The listing builds one solid part. Answer for the finished solid, in the listing's coordinates (mm). A direction names the side the tool comes from. Coordinates: 2 decimals unless noted, no trailing zeros. Loops run counter-clockwise (first coordinate to the right, second up) from the corner with the lowest first, then second, coordinate; pieces in that order, holes last. Notation, with made-up numbers: (-5, 83.5) - (12, 83.5) arc R25 cw to (12, 106.5) - close; hole circle Ø5 at (23.5, 25.5). An arc over 180 degrees is marked (long way). Put each result on its own line as item: value.
```python
from build123d import *

# Parameters (mm, degrees)
SKETCH2_R           = 1.6
CUT_EXTRUDE1_DEPTH  = 62.102373113
SKETCH8_R           = 10
CUT_EXTRUDE6_DEPTH  = 2
SKETCH16_R          = 1.5
CUT_EXTRUDE7_DEPTH  = 4
CUT_EXTRUDE10_DEPTH = 2


with BuildPart() as part:
    # Sketch1 → Revolve1 (revolve)
    with BuildSketch(Plane(origin=(0, 0, 0), x_dir=(0, 0, -1), z_dir=(1, 0, 0)), mode=Mode.PRIVATE) as revolve1_sk:
        Polygon((0, 0), (0, 42.5), (-3, 42.5), (-3, 19.55), (-3.5, 19.55), (-3.5, 17.55), (-11, 17.55), (-11, 0), align=None)
    revolve(revolve1_sk.sketch.rotate(Axis((0, 0, 11), (0, 0, -1)), 90), axis=Axis((0, 0, 11), (0, 0, -1)))

    # Sketch2 → Cut-Extrude1 (cut, through all)
    with BuildSketch(Plane(origin=(0, 0, 0), x_dir=(-1, 0, 0), z_dir=(0, 0, -1))):
        with Locations(Location((0, 36.75, 0), (0, 0, 90))):
            Circle(SKETCH2_R)
        with Locations(Location((36.75, 0, 0), (0, 0, 90))):
            Circle(SKETCH2_R)
        with Locations(Location((0, -36.75, 0), (0, 0, 90))):
            Circle(SKETCH2_R)
        with Locations(Location((-36.75, 0, 0), (0, 0, 90))):
            Circle(SKETCH2_R)
    extrude(amount=-CUT_EXTRUDE1_DEPTH, mode=Mode.SUBTRACT)

    # Sketch8 → Cut-Extrude6 (cut)
    with BuildSketch(Plane(origin=(0, 0, 0), x_dir=(-1, 0, 0), z_dir=(0, 0, -1))):
        Circle(SKETCH8_R)
    extrude(amount=-CUT_EXTRUDE6_DEPTH, mode=Mode.SUBTRACT)

    # Sketch16 → Cut-Extrude7 (cut)
    with BuildSketch(Plane(origin=(0, 0, 2), x_dir=(-1, 0, 0), z_dir=(0, 0, -1))):
        with Locations((4.065863992, 4.065863992)):
            Circle(SKETCH16_R)
        with Locations((-4.065863992, -4.065863992)):
            Circle(SKETCH16_R)
    extrude(amount=-CUT_EXTRUDE7_DEPTH, mode=Mode.SUBTRACT)

    # Sketch19 → Cut-Extrude10 (cut, symmetric)
    with BuildSketch(Plane(origin=(0, 0, 0), x_dir=(0, 0, 1), z_dir=(-0.7071067811865487, 0.7071067811865465, 0))):
        Polygon((0, -15), (0, 15), (1, 20), (1, 36), (0, 36), (0, 39), (3, 39), (3, 20), (2, 15), (2, -15), (3, -20), (3, -39), (0, -39), (0, -36), (1, -36), (1, -20), align=None)
    extrude(amount=CUT_EXTRUDE10_DEPTH, both=True, mode=Mode.SUBTRACT)


solid = part.part
```
1) Straight lines are drawn through the part: L1, parallel to Z at x = 12.5, y = 26.5; L2, parallel to Y at x = -4.5, z = 4.5; L3, parallel to Y at x = -11, z = 1. For each, find the intervals that lie inside material, in ascending order. Write a range as [from, to].
Found:
L1: z = [0, 3]
L2: y = [-16.96, 2.63], [5.5, 16.96]
L3: y = [-41.05, -13.83], [-8.17, 41.05]
2) The part is cut by section D-D (x = 7). Give the vertices of the cut face in (y, z), and give its area (3 significant figures).
Found:
outline: (-41.92, 0) - (-7.14, 0) - (-7.14, 2) - (9.83, 2) - (9.83, 0) - (41.92, 0) - (41.92, 3) - (18.25, 3) - (18.25, 3.5) - (16.09, 3.5) - (16.09, 11) - (-16.09, 11) - (-16.09, 3.5) - (-18.25, 3.5) - (-18.25, 3) - (-41.92, 3) - close
area: 477 mm^2
3) The part is cut by section C-C (y = -36.75). Give the vertices of the cut face in (x, z), and give its area (3 significant figures).
Found:
outline: (-21.35, 0) - (-1.6, 0) - (-1.6, 3) - (-21.35, 3) - close; (1.6, 0) - (21.35, 0) - (21.35, 3) - (1.6, 3) - close
area: 118 mm^2
4) Each of these flat-tipped pins is pushed along its axis until it touches: pin 1 (5 mm diameter, centred on x = -11.5, z = 6.5, fed in from +Y); pin 2 (11.5 mm diameter, centred on x = 17.5, y = 20.5, fed in from +Z); pin 3 (1.5 mm diameter, centred on x = 4.5, y = -4.5, fed in from -Z); pin 4 (10 mm diameter, centred on x = 1, y = -18.5, fed in from -Z). Where does it stop, or does it pass through?
Found:
pin 1: stops at y = 15.07
pin 2: stops at z = 3
pin 3: stops at z = 6
pin 4: stops at z = 0
5) For a pull along Y with two mould halves and no side action, classify faces 1 (the face through (18.65, -5.87, 3.25)), 2 (the face through (18, 9, 3)), 3 (the face through (-27.597, -27.557, 1.521)) as pulls with the +Y half, pulls with the -Y half, needs draft (parallel to the pull), parting line crosses it, or undercut.
Found:
face 1: parting line crosses it
face 2: needs draft
face 3: undercut
6) For faces 4 (the face through (12.379, 12.419, 2.507)), 5 (the face through (25.436, 25.476, 0.507)), 6 (the face through (-3.804, 17.133, 7.302)), 7 (the face through (-7.21, 6.93, 0.99)), determine the directions among +Z, -Z, +X, -X, +Y, -Y from which every point of the face is accessible in a straight line to the end or side of a thin tool.
Found:
face 4: none
face 5: +Z, -Z
face 6: +Z
face 7: -Z
7) The part is cut by section B-B (y = 0). Give the vertices of the cut face in (x, z), and give its area (3 significant figures).
Found:
outline: (-42.5, 0) - (-38.35, 0) - (-38.35, 3) - (-42.5, 3) - close; (-35.15, 0) - (-10, 0) - (-10, 2) - (10, 2) - (10, 0) - (35.15, 0) - (35.15, 3) - (19.55, 3) - (19.55, 3.5) - (17.55, 3.5) - (17.55, 11) - (-17.55, 11) - (-17.55, 3.5) - (-19.55, 3.5) - (-19.55, 3) - (-35.15, 3) - close; (38.35, 0) - (42.5, 0) - (42.5, 3) - (38.35, 3) - close
area: 479 mm^2
8) The part is cut by section A-A (x = -28). Give the vertices of the cut face in (y, z), and give its area (3 significant figures).
Found:
outline: (-31.97, 0) - (-27.15, 0) - (-27.15, 3) - (-31.97, 3) - close; (-25.17, 0) - (31.97, 0) - (31.97, 3) - (-25.17, 3) - close
area: 186 mm^2
